Work out the finished part from the listing and answer in its coordinate system (mm). Face numbers are marked on the shaded views. A direction names the side the tool comes from. Coordinates: 2 decimals unless noted, no trailing zeros. Order: outer loops, then holes, each group sorted by start corner. A loop starts at its lowest first (then second) coordinate and runs counter-clockwise, first axis right, second up. Notation, with made-up numbers: M 14,86.5 L 21,86.5 A24 cw 21,114.5 Z; hole C 5.5,87 d2. An arc over 180 degrees is marked long. Answer in a Markdown table with one row per item. Add a question column.
Item 1: The part is cut by section C-C (z = -0.25). Write down the section's boundary in (x, y), then the cut area to 3 significant figures.
Item 2: The part is cut by section A-A (y = 10.25). Write down the section's boundary in (x, z).
Item 3: The mould has two halves that part along X. Classify the marked faces 4, 5, 6 and 7: released by +X, released by -X, zero draft, split by the parting line, or undercut.
Item 4: The part is cut by section D-D (z = 1). Write down the section's boundary in (x, y), then the cut area to 3 significant figures.
Item 5: Which of the six approach directions +Z, -Z, +X, -X, +Y, -Y give full straight-line access (tool end or side, diameter ignored) to the marked faces 1, 2 and 3?
Item 6: The part is cut by section B-B (x = 0). Write down the section's boundary in (y, z), then the cut area to 3 significant figures.
Item 7: Flat-ended cylindrical pins translate along their axes: pin 1 Ø2.5 at (x, z) = (8, 2) entering from -Y; pin 2 Ø1.7 at (y, z) = (10, -1) entering from +X; pin 3 Ø0.8 at (y, z) = (2, -0.5) entering from +X; pin 4 Ø1.3 at (x, y) = (0.05, 6.78) entering from +Z. Find the tip coordinate at first contact, or state that the pin passes through.
Item 8: Consider line 1 (Z direction, x = 9.75, y = 5); line 2 (Y direction, x = 5.5, z = 1.25); line 3 (Z direction, x = 8, y = 6.25). Determine where each line is inside the solid, lowest interval first. Write a range as from..to.
Autodesk Inventor part; units mm, degrees
ref_plane "YZ Plane" through (0, 0, 0) normal (1, 0, 0) x (0, 1, 0)
ref_plane "XZ Plane" through (0, 0, 0) normal (0, 1, 0) x (-1, 0, 0)
ref_plane "XY Plane" through (0, 0, 0) normal (0, 0, 1) x (1, 0, 0)
sketch "Sketch1" plane through (0, 0, 0) normal (0, 0, 1) x (1, 0, 0)
  line L0 (4.9374, 6.4254) -> (10.2374, 6.4254) construction
  line L1 (4.9374, 4.0754) -> (10.2374, 4.0754)
  line L2 (10.2374, 8.7754) -> (4.9374, 8.7754)
  arc A0 (4.9374, 8.7754) -> (4.9374, 4.0754) centre (4.9374, 6.4254) ccw
  arc A1 (10.2374, 4.0754) -> (10.2374, 8.7754) centre (10.2374, 6.4254) ccw
  point P0 (0, 0)
  point P1 (7.5874, 6.4254)
  dimension "d0" = 10
  dimension "d1" = 4.7
extrude "Extrusion1" add sketch "Sketch1" along normal blind 7.3
fillet "Fillet1" radius 1 4 edges at (7.5874, 8.7754, 7.3) (2.5874, 6.4254, 7.3) (7.5874, 4.0754, 7.3) (12.5874, 6.4254, 7.3)
sketch "Sketch2" plane through (0, 0, 0) normal (0, 0, -1) x (-1, 0, 0)
  line L0 (-4.9374, 4.0754) -> (-10.2374, 4.0754)
  arc A0 (-4.9374, 4.0754) -> (-4.9374, 8.7754) centre (-4.9374, 6.4254) ccw
  line L1 (-10.2374, 8.7754) -> (-4.9374, 8.7754)
  arc A1 (-10.2374, 8.7754) -> (-10.2374, 4.0754) centre (-10.2374, 6.4254) ccw
  line L2 (-10.2374, 6.4254) -> (-4.9374, 6.4254) construction
  line L3 (-10.2374, 3.5754) -> (-4.9374, 3.5754)
  line L4 (-4.9374, 9.2754) -> (-10.2374, 9.2754)
  arc A2 (-10.2374, 9.2754) -> (-10.2374, 3.5754) centre (-10.2374, 6.4254) ccw
  arc A3 (-4.9374, 3.5754) -> (-4.9374, 9.2754) centre (-4.9374, 6.4254) ccw
  point P0 (0, 0)
  point P1 (-7.5874, 6.4254)
  dimension "d5" = 0.5
extrude "Extrusion2" add sketch "Sketch2" along normal blind 1.54
sketch "Sketch3" plane through (0, 0, 0) normal (0, 0, -1) x (-1, 0, 0)
  line L0 (-4.9374, 4.0754) -> (-10.2374, 4.0754)
  arc A0 (-4.9374, 4.0754) -> (-4.9374, 8.7754) centre (-4.9374, 6.4254) ccw
  line L1 (-10.2374, 8.7754) -> (-4.9374, 8.7754)
  arc A1 (-10.2374, 8.7754) -> (-10.2374, 4.0754) centre (-10.2374, 6.4254) ccw
  line L2 (-10.2374, 6.4254) -> (-4.9374, 6.4254) construction
  line L3 (-10.2374, 3.6254) -> (-4.9374, 3.6254)
  line L4 (-4.9374, 9.2254) -> (-10.2374, 9.2254)
  arc A2 (-10.2374, 9.2254) -> (-10.2374, 3.6254) centre (-10.2374, 6.4254) ccw
  arc A3 (-4.9374, 3.6254) -> (-4.9374, 9.2254) centre (-4.9374, 6.4254) ccw
  point P0 (0, 0)
  point P1 (-7.5874, 6.4254)
extrude "Extrusion3" add sketch "Sketch3" along normal blind 1.54 contours L0 A1 L1 A0
sketch "Sketch4" plane through (0, 0, -1.54) normal (0, 0, -1) x (-1, 0, 0)
  line L0 (-4.9374, 9.2754) -> (-10.2374, 9.2754)
  arc A0 (-10.2374, 9.2754) -> (-10.2374, 3.5754) centre (-10.2374, 6.4254) ccw
  line L1 (-10.2374, 6.4254) -> (-7.6274, 6.4254)
  circle A1 centre (-7.6274, 6.4254) radius 1.3
  point P0 (0, 0)
  dimension "d10" = 2.61
  dimension "d11" = 2.6
extrude "Extrusion4" cut sketch "Sketch4" against normal blind 2.96
sketch "Sketch5" plane through (0, 0, -1.54) normal (0, 0, -1) x (-1, 0, 0)
  arc A0 (-4.9374, 3.5754) -> (-4.9374, 9.2754) centre (-4.9374, 6.4254) ccw
  line L0 (-4.9374, 9.2754) -> (-10.2374, 9.2754)
  circle A1 centre (-15.1574, 5.9754) radius 0.8
  arc A2 (-15.6111, 7.4051) -> (-14.6795, 7.3972) centre (-15.1574, 5.9754) ccw
  line L1 (-15.6111, 8.031) -> (-15.6271, 8.031)
  line L2 (-15.6111, 7.4051) -> (-15.6111, 10.4765)
  line L3 (-4.6841, 10.5736) -> (-4.6841, 9.2641)
  line L4 (-14.6795, 7.3972) -> (-14.6795, 9.4832)
  line L5 (-5.6379, 9.578) -> (-5.6379, 9.2754)
  line L6 (-10.2374, 3.5754) -> (-4.9374, 3.5754)
  line L7 (-15.6111, 10.4765) -> (-15.6111, 11.4765)
  line L8 (-15.6111, 11.4765) -> (-4.6841, 11.4765)
  line L9 (-4.6841, 11.4765) -> (-4.6841, 10.2108)
  line L10 (-14.6795, 9.4832) -> (-14.6795, 10.4832)
  line L11 (-14.6795, 10.4832) -> (-5.6379, 10.4832)
  line L12 (-5.6379, 10.4832) -> (-5.6379, 9.578)
  point P0 (0, 0)
  dimension "d15" = 1.6
  dimension "d34" = 1
  dimension "d39" = 0.7
extrude "Extrusion5" add sketch "Sketch5" against normal blind 1.54
sketch "Sketch6" plane through (0, 0, -1.54) normal (0, 0, -1) x (-1, 0, 0)
  line L0 (-10.2374, 3.5754) -> (-4.9374, 3.5754)
  arc A0 (-10.2374, 9.2754) -> (-10.2374, 3.5754) centre (-10.2374, 6.4254) ccw
  circle A1 centre (-0.0485, 6.7803) radius 0.8
  arc A2 (0.4175, 5.3545) -> (-0.5144, 5.3545) centre (-0.0485, 6.7803) ccw
  line L1 (0.4175, 5.3545) -> (0.4175, 2.2034)
  line L2 (-0.5144, 3.7394) -> (-0.5144, 5.3545)
  line L3 (-0.5144, 3.7394) -> (-0.5144, 3.1974)
  line L4 (-10.4904, 2.2016) -> (-10.4904, 3.5866)
  line L5 (-9.5364, 3.1974) -> (-9.5364, 3.5754)
  line L6 (-5.6379, 10.4832) -> (-5.6379, 9.2754)
  line L7 (0.4175, 2.2034) -> (0.4175, 1.2016)
  line L8 (0.4175, 1.2016) -> (-10.4904, 1.2016)
  line L9 (-10.4904, 1.2016) -> (-10.4904, 2.2016)
  line L10 (-0.5144, 3.1974) -> (-0.5144, 2.1974)
  line L11 (-0.5144, 2.1974) -> (-9.5364, 2.1974)
  line L12 (-9.5364, 2.1974) -> (-9.5364, 3.1974)
  point P0 (0, 0)
  point P1 (-1.5346, 6.984)
  dimension "d22" = 1.6
  dimension "d37" = 1
  dimension "d40" = 0.7
extrude "Extrusion6" add sketch "Sketch6" against normal blind 1.54
properties part number "button"
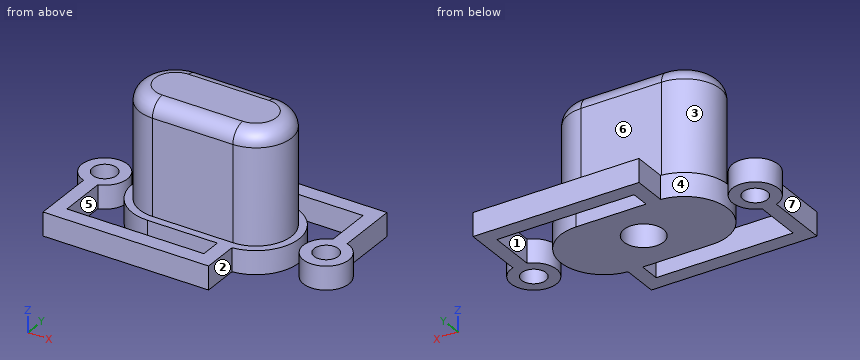
Reply:
| question | item | result |
|---|---|---|
| 1 | outline | M -0.42,1.2 L 10.49,1.2 L 10.49,3.59 A2.85 ccw 10.24,9.28 L 5.64,9.28 L 5.64,10.48 L 14.68,10.48 L 14.68,7.4 A1.5 ccw long 15.61,7.41 L 15.61,11.48 L 4.68,11.48 L 4.68,9.26 A2.85 ccw 4.94,3.58 L 9.54,3.58 L 9.54,2.2 L 0.51,2.2 L 0.51,5.35 A1.5 ccw long -0.42,5.35 Z; hole C 0.05,6.78 d1.6; hole C 7.63,6.43 d2.6; hole C 15.16,5.98 d1.6 |
| 1 | area | 90.4 mm2 |
| 2 | outline | M 4.68,-1.54 L 5.64,-1.54 L 5.64,0 L 4.68,0 Z; M 14.68,-1.54 L 15.61,-1.54 L 15.61,0 L 14.68,0 Z |
| 3 | face 4 | undercut |
| 3 | face 5 | undercut |
| 3 | face 6 | zero draft |
| 3 | face 7 | released by -X |
| 4 | outline | M 4.94,4.08 L 10.24,4.08 A2.35 ccw 10.24,8.78 L 4.94,8.78 A2.35 ccw Z; hole C 7.63,6.43 d2.6 |
| 4 | area | 37.0 mm2 |
| 5 | face 1 | +Z, -Z |
| 5 | face 2 | +Z, -Z, +X, -Y |
| 5 | face 3 | +Z, -X |
| 6 | outline | M 1.2,-1.54 L 5.98,-1.54 L 5.98,0 L 1.2,0 Z; M 7.58,-1.54 L 8.28,-1.54 L 8.28,0 L 7.58,0 Z |
| 6 | area | 8.44 mm2 |
| 7 | pin 1 | stops at y = 4.08 |
| 7 | pin 2 | stops at x = 15.61 |
| 7 | pin 3 | stops at x = 10.49 |
| 7 | pin 4 | passes through |
| 8 | line 1 | z = -1.54..7.3 |
| 8 | line 2 | y = 4.08..8.78 |
| 8 | line 3 | z = 1.42..7.3 |
